```python
from build123d import *

# Parameters (mm, degrees)
F0_W     = 120
F0_H     = 46
F1_DEPTH = 40


with BuildPart() as f1:
    # F0 (on Front) → F1 (new body, symmetric)
    with BuildSketch(Plane.XZ):
        Polygon((60, 0), (-60, 0), (-60, 150), (-62, 150), (-62, -150), (-60, -150), (-60, -50), (60, -50), (60, -150), (62, -150), (62, 150), (60, 150), align=None)
        with Locations((0, -25)):
            Rectangle(F0_W, F0_H, mode=Mode.SUBTRACT)
    extrude(amount=F1_DEPTH, both=True)


solid = f1.part
```
CAD build for the part. Positions are in the model's coordinates, mm. A direction names the side the tool comes from. Round coordinates to 2 decimals unless told otherwise and drop trailing zeros. Order: outer loops, then holes, each group sorted by start corner. A loop starts at its lowest first (then second) coordinate and runs counter-clockwise, first axis right, second up. Notation, with made-up numbers: (1.5, 54) -> (48.5, 54) arc R21 ccw to (48.5, 70) -> close; hole circle Ø5 at (-30, -32.75). An arc over 180 degrees is marked (long way). One line per question, with ' | ' between items.
Q1. Drop flat-ended pins along their axis: pin 1 (24 mm diameter, centred on x = -19, y = 11.5, fed in from -Z); pin 2 (2 mm diameter, centred on x = 10.5, y = -5.5, fed in from +Z). Give the stop position or say it passes through.
Completed:
pin 1: stops at z = -50 | pin 2: stops at z = 0
Q2. Which spindle directions (+Z, -Z, +X, -X, +Y, -Y) get a long thin tool onto all of the face, cutting with end or side? Do faces 1 (the flat face through (60, -1, 76)), 2 (the flat face through (-60, -1, -25)), 3 (the flat face through (62, -1, -2)), 4 (the flat face through (60, -1, -99)), 5 (the flat face through (-62, -1, 2)). Say none if no direction does.
Completed:
face 1: +Z, +Y, -Y | face 2: +Y, -Y | face 3: +Z, -Z, +X, +Y, -Y | face 4: -Z, +Y, -Y | face 5: +Z, -Z, -X, +Y, -Y
Q3. Slice it at B-B (z = -65). Write the cut outline in (x, y), then the cut area to 3 significant figures.
Completed:
outline: (-62, -40) -> (-60, -40) -> (-60, 40) -> (-62, 40) -> close; (60, -40) -> (62, -40) -> (62, 40) -> (60, 40) -> close | area: 320 mm^2
Q4. Two-plate mould, pull along Z, no slides. Class faces 6 (the flat face through (-1, -1, -2)), 7 (the flat face through (-1, -1, -50)), 8 (the flat face through (1, -1, 0)), 9 (the flat face through (-60, -1, -101)): released by +Z, released by -Z, zero draft, split by the parting line, or undercut.
Completed:
face 6: undercut | face 7: released by -Z | face 8: released by +Z | face 9: zero draft
Q5. Slice it at C-C (y = 7.5). Write the cut outline in (x, z).
Completed:
outline: (-62, -150) -> (-60, -150) -> (-60, -50) -> (60, -50) -> (60, -150) -> (62, -150) -> (62, 150) -> (60, 150) -> (60, 0) -> (-60, 0) -> (-60, 150) -> (-62, 150) -> close; hole (-60, -48) -> (60, -48) -> (60, -2) -> (-60, -2) -> close
Q6. Slice it at A-A (x = 6.5). Write the cut outline in (y, z).
Completed:
outline: (-40, -50) -> (40, -50) -> (40, -48) -> (-40, -48) -> close; (-40, -2) -> (40, -2) -> (40, 0) -> (-40, 0) -> close
Q7. Probe probe 1 along X at (y, z) = (-12, -4); probe 2 along Z at (x, y) = (-27, 32.5). List the from-to ranges inside material, lowest first.
Completed:
probe 1: x = -62 to -60, 60 to 62 | probe 2: z = -50 to -48, -2 to 0
